Read the model definition and answer for the solid it produces. Units are mm, in the model's axes. Face numbers are marked on the shaded views. Give positions to 0.01 mm unless a question says otherwise; leave off trailing zeros. Order: outer loops, then holes, each group sorted by start corner. A loop starts at its lowest first (then second) coordinate and runs counter-clockwise, first axis right, second up.
Item 1: Find the intervals of material crossed by line 1 along Y through (x, z) = (0, -1.75); line 2 along Y through (x, z) = (-5, -0.5); line 3 along X through (y, z) = (14.5, 10.25), in increasing order.
Item 2: The mould has two halves that part along Y. Classify the marked faces 1, 2, 3 and 4: +Y half, -Y half, draft (parallel to the pull), parting line (faces both ways), or undercut.
Item 3: A cutting plane is placed at B-B (x = -5.75). Write down the section's boundary in (y, z), plus the area to 3 significant figures.
Item 4: A cutting plane is placed at A-A (y = 12.7). Write down the section's boundary in (x, z), plus the area to 3 significant figures.
Item 5: Given pin 1 Ø3 at (y, z) = (18.5, -0.5) entering from +X; pin 2 Ø4 at (y, z) = (17.5, -7.5) entering from +X; pin 3 Ø1 at (x, z) = (3.5, -8.5) entering from +Y, each flat-ended and moving along its own axis, determine where each tip first touches the part or whether it passes through.
Item 6: A cutting plane is placed at D-D (y = 23.5). Write down the section's boundary in (x, z).
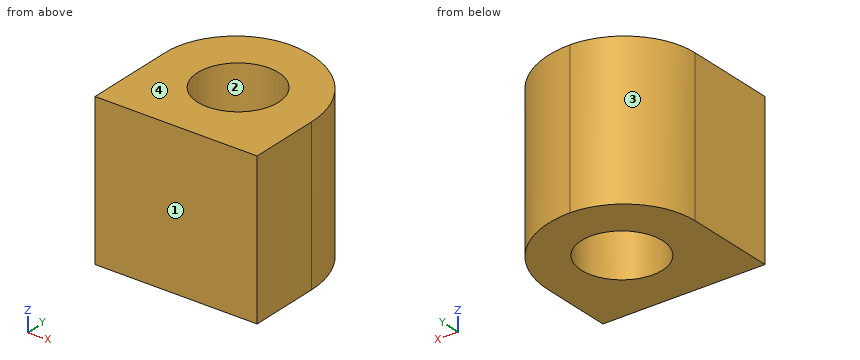
Autodesk Inventor part; units mm, degrees
ref_plane "YZ Plane" through (0, 0, 0) normal (1, 0, 0) x (0, 1, 0)
ref_plane "XZ Plane" through (0, 0, 0) normal (0, 1, 0) x (-1, 0, 0)
ref_plane "XY Plane" through (0, 0, 0) normal (0, 0, 1) x (1, 0, 0)
sketch "Sketch1" plane through (0, 0, 0) normal (0, 1, 0) x (-1, 0, 0)
  line L0 (-12.7, 11.9062) -> (12.7, 11.9062)
  line L1 (12.7, 11.9062) -> (12.7, -11.9062)
  line L2 (12.7, -11.9062) -> (-12.7, -11.9062)
  line L3 (-12.7, -11.9062) -> (-12.7, 11.9062)
  point P0 (0, 0)
  point P1 (-12.7, 0)
  point P2 (0, 11.9062)
  dimension "d0" = 25.4
  dimension "d1" = 23.8125
extrude "Extrusion1" add sketch "Sketch1" along normal blind 25.4
sketch "Sketch2" plane through (-12.7, 0, 11.9062) normal (0, 0, 1) x (1, 0, 0)
  circle A0 centre (12.7, 12.7) radius 6.35
  line L0 (0, 0) -> (0, 25.4)
  line L1 (25.4, 0) -> (0, 0)
  point P0 (12.7, 0)
  point P1 (0, 12.7)
  point P2 (12.7, 0)
  dimension "d4" = 12.7
extrude "Extrusion2" cut sketch "Sketch2" against normal blind 50.8
fillet "Fillet1" radius 14.2875 1 edges at (12.7, 25.4, 0)
fillet "Fillet2" radius 11.1125 1 edges at (-12.7, 25.4, 0)
properties part number "Gounded Clevis"
Response values:
1. line 1: y = 0 to 6.35, 19.05 to 25.31
1. line 2: y = 0 to 8.79, 16.61 to 24.86
1. line 3: x = -12.7 to -6.09, 6.09 to 12.29
2. face 1: -Y half
2. face 2: undercut
2. face 3: +Y half
2. face 4: draft
3. outline: (0, -11.91) - (10.01, -11.91) - (10.01, 11.91) - (0, 11.91) - close; (15.39, -11.91) - (24.59, -11.91) - (24.59, 11.91) - (15.39, 11.91) - close
3. area: 457 mm2
4. outline: (-12.7, -11.91) - (-6.35, -11.91) - (-6.35, 11.91) - (-12.7, 11.91) - close; (6.35, -11.91) - (12.61, -11.91) - (12.61, 11.91) - (6.35, 11.91) - close
4. area: 300 mm2
5. pin 1: stops at x = 11.43
5. pin 2: stops at x = 12.01
5. pin 3: stops at y = 24.64
6. outline: (-7.8, -11.91) - (5.53, -11.91) - (5.53, 11.91) - (-7.8, 11.91) - close
